Design review of the part built by this model. Coordinates are the model's own, in mm. Round coordinates to 2 decimals unless told otherwise and drop trailing zeros. Write each loop counter-clockwise with the first axis right and the second up, starting at its lowest first coordinate (ties: lowest second). Pieces come first, ordered by that corner, then holes. Notation, with made-up numbers: (65.5, 25.5) -> (81.5, 25.5) arc R22 ccw to (81.5, 59.5) -> close; hole circle Ø9 at (67.5, 0). An arc over 180 degrees is marked (long way). One line per question, with ' | ' between items. Start each with the question number.
1) Consider section B-B (x = -128.5). Give the boundary of the cut face in (y, z) (3 decimals).
2) Consider section A-A (z = 0.6). Give the boundary of the cut face in (x, y), then the cut area to 3 significant figures.
3) Consider section C-C (y = 142.5). Give the boundary of the cut face in (x, z) (3 decimals), then the cut area to 3 significant figures.
4) For probe 1 along Y at (x, z) = (-6.5, 3); probe 2 along X at (y, z) = (144, 2); probe 3 along X at (y, z) = (-154.5, 2.7), list the stretches that pass through material, from the lowest coordinate up.
5) Insertion check: pin 1 Ø10 at (x, y) = (91, -126) entering from -Z. The pin has a flat end and moves straight along its axis. Give the tip position at first contact, or say it passes through.
```python
from build123d import *

# Parameters (mm, degrees)
F1_DEPTH = 3.175


with BuildPart() as f1:
    # F0 (on Top) → F1 (new body)
    with BuildSketch(Plane.XY):
        Polygon((-18.594091, -184.605909), (169.170453, -76.2), (169.170453, 76.2), (-18.594091, 184.605909), (-150.576362, 108.405909), (-150.576362, -108.405909), align=None)
        Polygon((-31.294091, -191.938258), (-18.594091, -184.605909), (-150.576362, -108.405909), (-150.576362, -123.070606), align=None)
        Polygon((-150.576362, 108.405909), (-18.594091, 184.605909), (-31.294091, 191.938258), (-150.576362, 123.070606), align=None)
        Polygon((169.170453, 76.2), (169.170453, -76.2), (181.870453, -68.867652), (181.870453, 68.867652), align=None)
    extrude(amount=F1_DEPTH)


solid = f1.part
```
From the geometry:
1) outline: (-135.816, 0) -> (135.816, 0) -> (135.816, 3.175) -> (-135.816, 3.175) -> close
2) outline: (-150.58, -123.07) -> (-31.29, -191.94) -> (181.87, -68.87) -> (181.87, 68.87) -> (-31.29, 191.94) -> (-150.58, 123.07) -> close | area: 93,200 mm2
3) outline: (-116.924, 0) -> (54.335, 0) -> (54.335, 3.175) -> (-116.924, 3.175) -> close | area: 544 mm2
4) probe 1: y = -177.62 to 177.62 | probe 2: x = -114.33 to 51.74 | probe 3: x = -96.14 to 33.55
5) pin 1: stops at z = 0
